Verification items for the finished model (mm, model axes). Coordinates: 2 decimals unless noted, no trailing zeros. Order: outer loops, then holes, each group sorted by start corner. A loop starts at its lowest first (then second) coordinate and runs counter-clockwise, first axis right, second up.
Q1. Cross-section at C-C, the plane y = 0.6. Count the separate pieces of the cut face and the enclosed holes in it, and give its area (3 significant figures).
Q2. Thickness scan on line 1 (Z direction, x = 0, y = 0.9); line 2 (Z direction, x = 87, y = 2.25); line 3 (Z direction, x = -72.5, y = 2.45). Record the ranges inside material, lowest first.
Q3. Cross-section at A-A, the plane x = 0.5. Record the boundary of the cut face in (y, z).
Q4. Cross-section at D-D, the plane x = 87. Record the boundary of the cut face in (y, z), and give its area (3 significant figures).
Q5. Cross-section at B-B, the plane z = -10.5. Record the boundary of the cut face in (x, y).
Q6. Depth check by flat-ended pin: P1, Ø1.5, axis at y = 1.5, z = -7.5, coming from the +X side; P2, Ø1.5, axis at x = 2, y = 1, coming from the +Z side; P3, Ø1.5, axis at y = 1, z = -54.5, coming from the +X side; P4, Ø1, axis at y = 2.5, z = -92, coming from the +X side. Enter the tip coordinate at first touch or a pass-through.
from build123d import *

# Parameters (mm, degrees)
BOSS_EXTRUDE1_DEPTH = 3
SKETCH2_W           = 10
SKETCH2_H           = 3
CUT_EXTRUDE3_DEPTH  = 10


with BuildPart() as part:
    # Sketch1 → Boss-Extrude1 (new body)
    with BuildSketch(Plane(origin=(0, 0, 0), x_dir=(1, 0, 0), z_dir=(0, 1, 0))):
        Polygon((-123, 0), (123, 0), (123, 38), (52.5, 168), (-52.5, 168), (-123, 38), align=None)
    extrude(amount=BOSS_EXTRUDE1_DEPTH)

    # Sketch2 → Cut-Extrude3 (cut)
    with BuildSketch(Plane(origin=(0, 3, 0), x_dir=(1, 0, 0), z_dir=(0, 1, 0))):
        Polygon((120, 3), (120, 0), (123, 0), (123, 14), (120, 14), align=None)
        Polygon((120, 37.23889635), (120, 24), (123, 24), (123, 38), (105.456749613, 70.349256033), (102.819582002, 68.919099751), align=None)
        Polygon((70.539591859, 128.44248583), (98.052394397, 77.709658456), (100.689562008, 79.139814737), (73.17675947, 129.872642111), align=None)
        Polygon((50.714170713, 165), (65.772404254, 137.233044534), (68.409571865, 138.663200816), (52.5, 168), (49.087247636, 168), align=None)
        Polygon((14.314512119, 124.067092532), (11.385651621, 123.417649552), (9.220841688, 133.180517879), (12.149702186, 133.829960859), align=None)
        Polygon((-12.149702186, 133.829960859), (-14.314512119, 124.067092532), (-11.385651621, 123.417649552), (-9.220841688, 133.180517879), align=None)
        with Locations((0, 54.5)):
            Rectangle(SKETCH2_W, SKETCH2_H)
        Polygon((-52.5, 168), (-68.409571865, 138.663200816), (-65.772404254, 137.233044534), (-50.714170713, 165), (-49.087247636, 168), align=None)
        Polygon((-73.17675947, 129.872642111), (-100.689562008, 79.139814737), (-98.052394397, 77.709658456), (-70.539591859, 128.44248583), align=None)
        Polygon((-123, 14), (-123, 0), (-120, 0), (-120, 3), (-120, 14), align=None)
        Polygon((-123, 38), (-123, 24), (-120, 24), (-120, 37.23889635), (-102.819582002, 68.919099751), (-105.456749613, 70.349256033), align=None)
    extrude(amount=-CUT_EXTRUDE3_DEPTH, mode=Mode.SUBTRACT)


solid = part.part
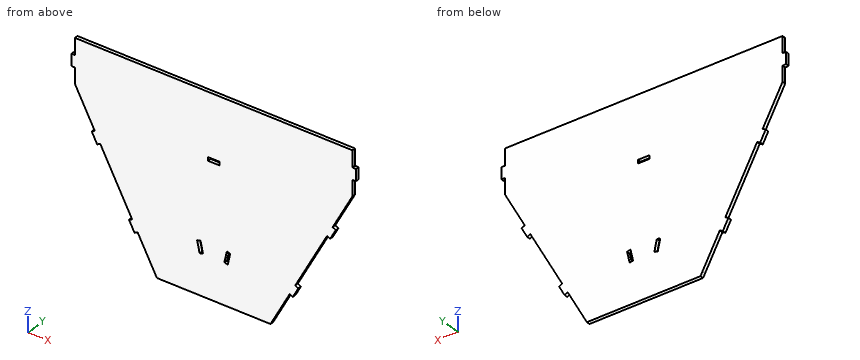
Check values:
1. separate pieces: 1
1. enclosed holes: 3
1. area: 31,100 mm2
2. line 1: z = -168 to -56, -53 to 0
2. line 2: z = -98.09 to 0
2. line 3: z = -131.12 to -129.51, -124.83 to 0
3. outline: (0, -168) - (3, -168) - (3, -56) - (0, -56) - close; (0, -53) - (3, -53) - (3, 0) - (0, 0) - close
4. outline: (0, -98.09) - (3, -98.09) - (3, 0) - (0, 0) - close
4. area: 294 mm2
5. outline: (-120, 0) - (120, 0) - (120, 3) - (-120, 3) - close
6. P1: stops at x = 120
6. P2: stops at z = 0
6. P3: stops at x = 111.05
6. P4: stops at x = 90.57
